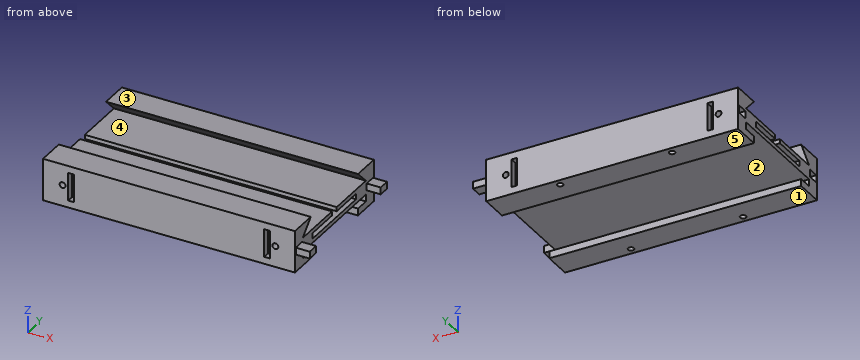
```python
from build123d import *

# Parameters (mm, degrees)
F0_W      = 180
F0_H      = 100
F1_DEPTH  = 30
F3_DEPTH  = 180
F4_W      = 8
F4_H      = 5
F5_DEPTH  = 10
F6_W      = 8.3
F6_H      = 5.3
F7_DEPTH  = 10.2
F8_W      = 4
F8_H      = 20
F9_DEPTH  = 5
F10_W     = 4
F10_H     = 20
F11_DEPTH = 5
F12_D     = 4.2
F12_DEPTH = 10
F12_TIP   = 1.2618073
F13_D     = 4.2
F13_DEPTH = 10
F13_TIP   = 1.2618073
F15_D     = 4.2
F15_DEPTH = 7.6
F15_TIP   = 1.2618073


with BuildPart() as f1:
    # F0 (on Top) → F1 (new body)
    with BuildSketch(Plane.XY):
        Rectangle(F0_W, F0_H)
    extrude(amount=F1_DEPTH)

    # F2 (on face) → F3 (cut)
    with BuildSketch(Plane.YZ.offset(90)):
        Polygon((30, 30), (-30, 30), (-40, 20), (-3, 20), (3, 20), (40, 20), align=None)
        Polygon((-30, 5), (-30, 0), (30, 0), (30, 5), (40, 5), (40, 10), (-40, 10), (-40, 5), align=None)
        Polygon((3, 20), (-3, 20), (-3, 17), (-27.5, 17), (-27.5, 13), (27.5, 13), (27.5, 17), (3, 17), align=None)
    extrude(amount=-F3_DEPTH, mode=Mode.SUBTRACT)

    # F4 (on face) → F5 (join)
    with BuildSketch(Plane.YZ.offset(90)):
        with Locations((-45, 15)):
            Rectangle(F4_W, F4_H)
        with Locations((45, 15)):
            Rectangle(F4_W, F4_H)
    extrude(amount=F5_DEPTH)

    # F6 (on face) → F7 (cut)
    with BuildSketch(Plane(origin=(-90, 0, 0), x_dir=(0, -1, 0), z_dir=(-1, 0, 0))):
        with Locations((-45, 15)):
            Rectangle(F6_W, F6_H)
        with Locations((45, 15)):
            Rectangle(F6_W, F6_H)
    extrude(amount=-F7_DEPTH, mode=Mode.SUBTRACT)

    # F8 (on face) → F9 (cut)
    with BuildSketch(Plane.XZ.offset(50)):
        with Locations((-70, 15)):
            Rectangle(F8_W, F8_H)
        with Locations((70, 15)):
            Rectangle(F8_W, F8_H)
    extrude(amount=-F9_DEPTH, mode=Mode.SUBTRACT)

    # F10 (on face) → F11 (cut)
    with BuildSketch(Plane(origin=(0, 50, 0), x_dir=(-1, 0, 0), z_dir=(0, 1, 0))):
        with Locations((70, 15)):
            Rectangle(F10_W, F10_H)
        with Locations((-70, 15)):
            Rectangle(F10_W, F10_H)
    extrude(amount=-F11_DEPTH, mode=Mode.SUBTRACT)

    # F12
    with Locations(Plane.XZ.offset(50)):
        with Locations((-76, 15), (76, 15)):
            Hole(F12_D / 2, depth=F12_DEPTH)
            with Locations((0, 0, -(F12_DEPTH + F12_TIP / 2))):  # 118° drill point
                Cone(0, F12_D / 2, F12_TIP, mode=Mode.SUBTRACT)

    # F13
    with Locations(Plane(origin=(0, 50, 0), x_dir=(-1, 0, 0), z_dir=(0, 1, 0))):
        with Locations((-76, 15), (76, 15)):
            Hole(F13_D / 2, depth=F13_DEPTH)
            with Locations((0, 0, -(F13_DEPTH + F13_TIP / 2))):  # 118° drill point
                Cone(0, F13_D / 2, F13_TIP, mode=Mode.SUBTRACT)

    # F15
    with Locations(Plane(origin=(0, 0, 0), x_dir=(1, 0, 0), z_dir=(0, 0, -1))):
        with Locations((-40, 45), (40, 45), (40, -45), (-40, -45)):
            Hole(F15_D / 2, depth=F15_DEPTH)
            with Locations((0, 0, -(F15_DEPTH + F15_TIP / 2))):  # 118° drill point
                Cone(0, F15_D / 2, F15_TIP, mode=Mode.SUBTRACT)


solid = f1.part
```
Can you work these out from the model? Positions are in its coordinate system, mm. Face numbers are marked on the shaded views. A direction names the side the tool comes from. Coordinates: 2 decimals unless noted, no trailing zeros. Order: outer loops, then holes, each group sorted by start corner. A loop starts at its lowest first (then second) coordinate and runs counter-clockwise, first axis right, second up. Notation, with made-up numbers: (2.25, 27.25) - (13.25, 27.25) arc R16 cw to (13.25, 51.25) - close; hole circle Ø3 at (22, 2). An arc over 180 degrees is marked (long way). Answer in a Markdown table with one row per item.
1. For pin 1 (2.5 mm diameter, centred on x = 76, z = 15, fed in from +Y); pin 2 (6 mm diameter, centred on y = 8, z = 21.5, fed in from +X); pin 3 (8 mm diameter, centred on x = 52, y = 9, fed in from -Z), each with a flat end and sliding along its axis, tell me the tip position at first contact or that it passes through.
Reply:
| item | result |
|---|---|
| pin 1 | stops at y = 39.49 |
| pin 2 | stops at x = 90 |
| pin 3 | stops at z = 10 |
2. For the marked faces 1 and 2, which set-ups out of +Z, -Z, +X, -X, +Y, -Y let a thin tool reach every point of the face, with its end or its side?
Reply:
| item | result |
|---|---|
| face 1 | -Z, +X, -X, +Y, -Y |
| face 2 | +X, -X |
3. If I drill on line 1 along X through (y, z) = (-44, 15); line 2 along Y through (x, z) = (-40, 6.25); line 3 along X through (y, z) = (-45, 3), over which ranges is the centre line in solid material (lowest first)?
Reply:
| item | result |
|---|---|
| line 1 | x = -79.8 to -78.1, -73.9 to 73.9, 78.1 to 100 |
| line 2 | y = -50 to -47.1, -42.9 to -40, 40 to 42.9, 47.1 to 50 |
| line 3 | x = -90 to -42.1, -37.9 to 37.9, 42.1 to 90 |
4. Suppose I cut it at B-B (x = -0.5). Please give me the cut outline in (y, z).
Reply:
| item | result |
|---|---|
| outline | (-50, 0) - (-30, 0) - (-30, 5) - (-40, 5) - (-40, 10) - (40, 10) - (40, 5) - (30, 5) - (30, 0) - (50, 0) - (50, 30) - (30, 30) - (40, 20) - (3, 20) - (3, 17) - (27.5, 17) - (27.5, 13) - (-27.5, 13) - (-27.5, 17) - (-3, 17) - (-3, 20) - (-40, 20) - (-30, 30) - (-50, 30) - close |
5. If we mould it in two halves opening along Z, with no side actions, what happens to the marked faces 3, 4 and 5? For each: pulls with the +Z half, pulls with the -Z half, needs draft (parallel to the pull), parting line crosses it, or undercut.
Reply:
| item | result |
|---|---|
| face 3 | pulls with the +Z half |
| face 4 | undercut |
| face 5 | pulls with the -Z half |
6. Suppose I cut it at A-A (y = -12). Please give me the cut outline in (x, z), and give its area (3 significant figures).
Reply:
| item | result |
|---|---|
| outline | (-90, 10) - (90, 10) - (90, 13) - (-90, 13) - close; (-90, 17) - (90, 17) - (90, 20) - (-90, 20) - close |
| area | 1,080 mm^2 |
